Read the model definition and answer for the solid it produces. Units are mm, in the model's axes. Face numbers are marked on the shaded views. A direction names the side the tool comes from. Give positions to 0.01 mm unless a question says otherwise; leave off trailing zeros. Loops run counter-clockwise (first coordinate to the right, second up) from the corner with the lowest first, then second, coordinate; pieces in that order, holes last. Notation, with made-up numbers: (54, -38) - (96, -38) arc R8 ccw to (96, -30) - close; hole circle Ø4 at (80, 52.5). An arc over 180 degrees is marked (long way). Write item = value, one per line. Start each with the question number.
from build123d import *

# Parameters (mm, degrees)
F1_DEPTH = 63.5
F0_W     = 25.4
F0_H     = 19.05
F2_DEPTH = 25.4
F3_DEPTH = 7.9375
F5_R     = 6.35


with BuildPart() as f1:
    # F0 (on Front) → F1 (new body, symmetric)
    with BuildSketch(Plane.XZ):
        Polygon((-41.275, 9.525), (-41.275, -9.525), (41.275, -9.525), (41.275, 9.525), (22.225, 9.525), align=None)
    extrude(amount=F1_DEPTH, both=True)

    # F0 (on Front) → F2 (join, symmetric)
    with BuildSketch(Plane.XZ):
        with BuildLine():
            Line((22.225, 9.525), (41.275, 9.525))
            Line((41.275, 9.525), (41.275, 27.234414))
            ThreePointArc((41.275, 27.234414), (46.930285, 39.382379), (59.86688, 42.8752))
            Line((59.86688, 42.8752), (68.073841, 42.8752))
            Line((68.073841, 42.8752), (68.073841, 61.9252))
            add(Edge.make_bspline(
                [(49.186449, 61.239376), (55.109251, 61.677968), (61.396661, 61.911853), (68.073841, 61.9252)],
                knots=[109.362074, 109.362074, 109.362074, 109.362074, 121.255722, 121.255722, 121.255722, 121.255722], degree=3))
            ThreePointArc((49.186449, 61.239376), (29.783208, 48.93267), (22.225, 27.234414))
            Line((22.225, 27.234414), (22.225, 9.525))
        make_face()
        with Locations((80.773841, 52.4002)):
            Rectangle(F0_W, F0_H)
    extrude(amount=F2_DEPTH, both=True)

    # F0 (on Front) → F3 (join, symmetric)
    with BuildSketch(Plane.XZ):
        with BuildLine():
            add(Edge.make_bspline(
                [(-41.275, 9.525), (-28.906992, 35.866078), (-5.273707, 57.206524), (49.186449, 61.239376)],
                knots=[0, 0, 0, 0, 109.362074, 109.362074, 109.362074, 109.362074], degree=3))
            Line((-41.275, 9.525), (22.225, 9.525))
            Line((22.225, 9.525), (22.225, 27.234414))
            ThreePointArc((22.225, 27.234414), (29.783208, 48.93267), (49.186449, 61.239376))
        make_face()
    extrude(amount=F3_DEPTH, both=True)

    # F0 (on Front) → F4 (revolve)
    with BuildSketch(Plane.XZ):
        Polygon((93.473841, 66.675), (93.473841, 61.9252), (93.473841, 42.8752), (93.473841, 38.1), (118.873841, 38.1), (118.873841, 66.675), align=None)
    revolve(axis=Axis((93.473841, 0, 52.3875), (0, 0, 1)))

    # F5
    f5_edges = [f1.edges().sort_by_distance(p)[0] for p in [
        (-41.275, -63.5, 0),
        (41.275, -63.5, 0),
        (41.275, 63.5, 0),
        (-41.275, 63.5, 0),
    ]]
    fillet(f5_edges, radius=F5_R)


solid = f1.part
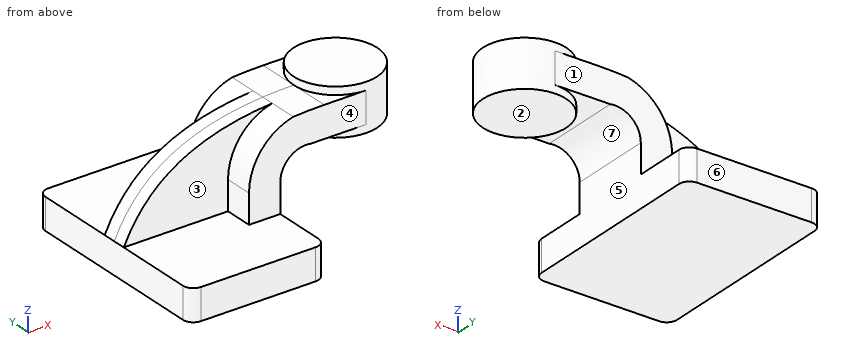
1. A cutting plane is placed at B-B on y = -44.5. Give the vertices of the cut face in (x, z) (3 decimals).
2. A tool of negligible diameter and unlimited length cuts with its end or side. For the marked faces 1, 2, 3 and 4, from which of +Z, -Z, +X, -X, +Y, -Y can it reach the whole face along a straight path? Write none if from no direction.
3. A cutting plane is placed at A-A on z = -4. Give the vertices of the cut face in (x, y) (3 decimals).
4. A cutting plane is placed at C-C on x = 79. Give the vertices of the cut face in (y, z) (3 decimals).
5. Given P1, Ø16.5, axis at x = -15, y = -25, coming from the +Z side (3 decimals); P2, Ø5, axis at y = 19.5, z = 14.5, coming from the -X side (3 decimals); P3, Ø2, axis at x = 94, y = -3, coming from the -Z side, each flat-ended and moving along its own axis, determine where each tip first touches the part or whether it passes through.
6. For a pull along X with two mould halves and no side action, classify the marked faces 5, 6 and 7 as released by +X, released by -X, zero draft, split by the parting line, or undercut.
7. Consider line 1 along Y through (x, z) = (25.5, 45); line 2 along Z through (x, y) = (-24.5, 15) (3 decimals); line 3 along X through (y, z) = (1.5, 3) (3 decimals). Determine where each line is inside the solid, lowest interval first. Write a range as [from, to].
Reply:
q1.outline = (-41.275, -9.525) - (41.275, -9.525) - (41.275, 9.525) - (-41.275, 9.525) - close
q2.face_1 = +Z, +X, -X, +Y
q2.face_2 = -Z, +X, +Y, -Y
q2.face_3 = +Z, -X, -Y
q2.face_4 = +Z, +X, -X, -Y
q3.outline = (-41.275, -57.15) arc R6.35 ccw to (-34.925, -63.5) - (34.925, -63.5) arc R6.35 ccw to (41.275, -57.15) - (41.275, 57.15) arc R6.35 ccw to (34.925, 63.5) - (-34.925, 63.5) arc R6.35 ccw to (-41.275, 57.15) - close
q4.outline = (-25.4, 42.875) - (-20.873, 42.875) - (-20.873, 38.1) - (20.873, 38.1) - (20.873, 42.875) - (25.4, 42.875) - (25.4, 61.925) - (20.873, 61.925) - (20.873, 66.675) - (-20.873, 66.675) - (-20.873, 61.925) - (-25.4, 61.925) - close
q5.P1 = 9.525
q5.P2 = 22.225
q5.P3 = 38.1
q6.face_5 = released by +X
q6.face_6 = zero draft
q6.face_7 = undercut
q7.line_1 = [-7.94, 7.94]
q7.line_2 = [-9.525, 9.525]
q7.line_3 = [-41.275, 41.275]
